from build123d import *

# Parameters (mm, degrees)
F1_W      = 20
F1_H      = 300
F2_DEPTH  = 200
F0_W      = 200
F0_H      = 300
F3_DEPTH  = 1.5
F4_W      = 22.1463561058
F4_H      = 300
F5_DEPTH  = 200
F6_W      = 200
F6_H      = 300
F7_DEPTH  = 9
F8_W      = 200
F8_H      = 209
F9_DEPTH  = 25
F10_R     = 37.0701897266
F11_DEPTH = 25


with BuildPart() as f2:
    # F1 (on face) → F2 (new body)
    with BuildSketch(Plane.XZ):
        with Locations((10, 150)):
            Rectangle(F1_W, F1_H)
    extrude(amount=F2_DEPTH)

    # F0 (on Front) + F1 (on face) → F3 (join)
    with BuildSketch(Plane.XZ):
        with Locations((100, 150)):
            Rectangle(F0_W, F0_H)
    with BuildSketch(Plane.XZ):
        with Locations((10, 150)):
            Rectangle(F1_W, F1_H)
    extrude(amount=F3_DEPTH)

    # F4 (on face) → F5 (join)
    with BuildSketch(Plane.XZ.offset(1.5)):
        with Locations((188.9268219471, 150)):
            Rectangle(F4_W, F4_H)
    extrude(amount=F5_DEPTH)

    # F6 (on face) → F7 (join)
    with BuildSketch(Plane.XZ.offset(200)):
        with Locations((100, 150)):
            Rectangle(F6_W, F6_H)
    extrude(amount=F7_DEPTH)

    # F8 (on face) → F9 (join)
    with BuildSketch(Plane.XY.offset(300)):
        with Locations((100, -104.5)):
            Rectangle(F8_W, F8_H)
    extrude(amount=F9_DEPTH)

    # F10 (on face) → F11 (cut)
    with BuildSketch(Plane.XZ.offset(209)):
        with Locations((143.6603814363, 270.9373235703)):
            Circle(F10_R)
    extrude(amount=-F11_DEPTH, mode=Mode.SUBTRACT)


solid = f2.part
Geometry check sheet. Reference: the model listing, model coordinates, mm. A direction names the side the tool comes from. Give positions to 0.01 mm unless a question says otherwise; leave off trailing zeros. Write each loop counter-clockwise with the first axis right and the second up, starting at its lowest first coordinate (ties: lowest second). Pieces come first, ordered by that corner, then holes. Notation, with made-up numbers: M 55.25,12 L 99.25,12 A14 cw 99.25,16 Z; hole C 60,56.25 d1. An arc over 180 degrees is marked long. Answer as CSV lines item,"result". Start each with the question number.
Q1. Section check D-D, the plane x = 63.5. Record the cut outline in (y, z), then the cut area to 4 significant figures.
Q2. Release check for a two-part mould opening along X. For faces 1 (the face through (99, 0, 160)), 2 (the face through (0, -106, 160)), 3 (the face through (200, -106, 160)), 4 (the face through (163.589, -199.453, 302.195)) record: pulls with the +X half, pulls with the -X half, needs draft (parallel to the pull), parting line crosses it, or undercut.
Q3. Material ranges on L1, parallel to Y at x = 112.5, z = 108.5; L2, parallel to X at y = -145, z = 153; L3, parallel to Z at x = 119, y = -87.5, recorded low to high.
Q4. Go/stop test with a flat-tipped pin: pin 1 (1.5 mm diameter, centred on x = 104.5, y = -163, fed in from -Z). Record where the tip stops, or that it passes through.
Q5. Section check A-A, the plane z = 100. Record the cut outline in (x, y).
Q6. Section check C-C, the plane y = -195.5. Record the cut outline in (x, z), then the cut area to 3 significant figures.
Q7. Tool access check on faces 5 (the face through (143, -184, 303)), 6 (the face through (20, -99, 148)), 7 (the face through (18, -119, 0)). Record the directions out of +Z, -Z, +X, -X, +Y, -Y that give a thin tool (end or side, any length) a straight path to the whole face; none if there is none.
Q8. Section check B-B, the plane x = 114. Record the cut outline in (y, z), then the cut area to 3 significant figures.
Geometry says:
1,outline,"M -209,0 L -200,0 L -200,300 L -1.5,300 L -1.5,0 L 0,0 L 0,325 L -209,325 Z"
1,area,"8,375 mm^2"
2,face 1,"needs draft"
2,face 2,"pulls with the -X half"
2,face 3,"pulls with the +X half"
2,face 4,"undercut"
3,L1,"-209 to -200, -1.5 to 0"
3,L2,"0 to 20, 177.85 to 200"
3,L3,"300 to 325"
4,pin 1,"z = 300"
5,outline,"M 0,-209 L 200,-209 L 200,0 L 0,0 Z; hole M 20,-200 L 177.85,-200 L 177.85,-1.5 L 20,-1.5 Z"
6,outline,"M 0,0 L 20,0 L 20,300 L 120.65,300 A37.07 cw 166.67,300 L 177.85,300 L 177.85,285.26 A37.07 cw 177.85,256.62 L 177.85,0 L 200,0 L 200,325 L 0,325 Z"
6,area,"17,300 mm^2"
7,face 5,"-Z, -Y"
7,face 6,"-Z"
7,face 7,"-Z, +X, -X, +Y, -Y"
8,outline,"M -209,0 L -200,0 L -200,248.7 L -209,248.7 Z; M -209,293.17 L -200,293.17 L -200,300 L -1.5,300 L -1.5,0 L 0,0 L 0,325 L -209,325 Z"
8,area,"7,970 mm^2"
